from build123d import *

# Parameters (mm, degrees)
SKETCH1_W                 = 175
SKETCH1_H                 = 260
BOSS_EXTRUDE1_DEPTH       = 3
SKETCH3_W                 = 12.7
SKETCH3_H                 = 12.7
SKETCH3_W_2               = 8.7
SKETCH3_H_2               = 8.7
EXTRUDE_THIN1_DEPTH       = 328
MIRROR2_COPY_1_SKETCH_W   = 12.7
MIRROR2_COPY_1_SKETCH_H   = 12.7
MIRROR2_COPY_1_SKETCH_W_2 = 8.7
MIRROR2_COPY_1_SKETCH_H_2 = 8.7
MIRROR2_COPY_1_DEPTH      = 328
SKETCH5_W                 = 175
SKETCH5_H                 = 260
SKETCH5_W_2               = 171
SKETCH5_H_2               = 256
EXTRUDE_THIN2_DEPTH       = 83
SKETCH6_W                 = 175
SKETCH6_H                 = 260
BOSS_EXTRUDE2_DEPTH       = 2
SKETCH8_R                 = 22.5
CUT_EXTRUDE1_DEPTH        = 364.51100396
SKETCH9_R                 = 7.5
CUT_EXTRUDE2_DEPTH        = 3


with BuildPart() as part:
    # Sketch1 → Boss-Extrude1 (new body)
    with BuildSketch(Plane(origin=(0, 0, 0), x_dir=(1, 0, 0), z_dir=(0, 1, 0))):
        Rectangle(SKETCH1_W, SKETCH1_H)
    extrude(amount=BOSS_EXTRUDE1_DEPTH)

    # Sketch3 → Extrude-Thin1 (add)
    with BuildSketch(Plane(origin=(0, 3, 0), x_dir=(1, 0, 0), z_dir=(0, 1, 0))):
        with Locations((-81.15, 123.65)):
            Rectangle(SKETCH3_W, SKETCH3_H)
        with Locations((-81.15, 123.65)):
            Rectangle(SKETCH3_W_2, SKETCH3_H_2, mode=Mode.SUBTRACT)
    extrude_thin1 = extrude(amount=EXTRUDE_THIN1_DEPTH)

    # Mirror1: Extrude-Thin1 across plane
    add(extrude_thin1.mirror(Plane(origin=(0, 0, 0), x_dir=(0, 0, 1), z_dir=(1, 0, 0))))

    # Mirror2: Extrude-Thin1 across plane
    add(extrude_thin1.mirror(Plane.XY))

    # Mirror2 copy 1 sketch → Mirror2 copy 1 (add)
    with BuildSketch(Plane(origin=(0, 3, 0), x_dir=(-1, 0, 0), z_dir=(0, 1, 0))):
        with Locations((-81.15, 123.65)):
            Rectangle(MIRROR2_COPY_1_SKETCH_W, MIRROR2_COPY_1_SKETCH_H)
        with Locations((-81.15, 123.65)):
            Rectangle(MIRROR2_COPY_1_SKETCH_W_2, MIRROR2_COPY_1_SKETCH_H_2, mode=Mode.SUBTRACT)
    extrude(amount=MIRROR2_COPY_1_DEPTH)

    # Sketch5 → Extrude-Thin2 (add)
    with BuildSketch(Plane(origin=(0, 3, 0), x_dir=(1, 0, 0), z_dir=(0, 1, 0))):
        Rectangle(SKETCH5_W, SKETCH5_H)
        Rectangle(SKETCH5_W_2, SKETCH5_H_2, mode=Mode.SUBTRACT)
    extrude(amount=EXTRUDE_THIN2_DEPTH)

    # Sketch6 → Boss-Extrude2 (add)
    with BuildSketch(Plane(origin=(0, 86, 0), x_dir=(1, 0, 0), z_dir=(0, 1, 0))):
        Rectangle(SKETCH6_W, SKETCH6_H)
    extrude(amount=BOSS_EXTRUDE2_DEPTH)

    # Sketch8 → Cut-Extrude1 (cut, through all)
    with BuildSketch(Plane(origin=(0, 3, 0), x_dir=(1, 0, 0), z_dir=(0, 1, 0))):
        with Locations((0, -60)):
            Circle(SKETCH8_R)
        with BuildLine():
            ThreePointArc((22.5, 0), (0, -22.5), (-22.5, 0))
            Line((-22.5, 0), (-22.5, -60))
            ThreePointArc((-22.5, -60), (0, -37.5), (22.5, -60))
            Line((22.5, -60), (22.5, 0))
        make_face()
        Circle(SKETCH8_R)
    extrude(amount=CUT_EXTRUDE1_DEPTH, mode=Mode.SUBTRACT)

    # Sketch9 → Cut-Extrude2 (cut)
    with BuildSketch(Plane.XZ):
        with Locations((-15, -112.5)):
            Circle(SKETCH9_R)
        with BuildLine():
            Line((15, -105), (-15, -105))
            ThreePointArc((-15, -105), (-9.696699141, -107.196699141), (-7.5, -112.5))
            ThreePointArc((-7.5, -112.5), (-9.696699141, -117.803300859), (-15, -120))
            Line((-15, -120), (15, -120))
            ThreePointArc((15, -120), (7.5, -112.5), (15, -105))
        make_face()
        with Locations((15, -112.5)):
            Circle(SKETCH9_R)
    extrude(amount=-CUT_EXTRUDE2_DEPTH, mode=Mode.SUBTRACT)


solid = part.part
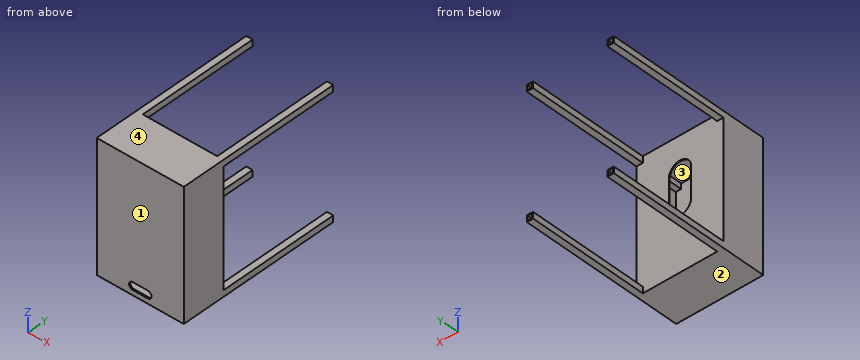
Geometry: final body of the model. Coordinates: model frame, mm. Face numbers are marked on the shaded views. Give positions to 0.01 mm unless a question says otherwise; leave off trailing zeros. Order: outer loops, then holes, each group sorted by start corner. A loop starts at its lowest first (then second) coordinate and runs counter-clockwise, first axis right, second up. Notation, with made-up numbers: (28.25, -33.75) -> (53.25, -33.75) arc R13 ccw to (53.25, -13.75) -> close; hole circle Ø1 at (-33, -2.75). An arc over 180 degrees is marked (long way). Write each question's results on one line, items separated by ' | '.
1) Cut plane D-D (z = 12). Output: boundary loops of the cut face in (x, y), and give its area (3 significant figures).
Geometry says:
outline: (-87.5, 0) -> (87.5, 0) -> (87.5, 88) -> (22.5, 88) -> (22.5, 86) -> (85.5, 86) -> (85.5, 3) -> (-85.5, 3) -> (-85.5, 86) -> (-22.5, 86) -> (-22.5, 88) -> (-87.5, 88) -> close | area: 1,120 mm²
2) Cut plane A-A (y = 110). Give the number of separate pieces and of enclosed holes in the cut face, and give its area (3 significant figures).
Geometry says:
separate pieces: 4 | enclosed holes: 4 | area: 342 mm²
3) Cut plane B-B (x = 0). Output: boundary loops of the cut face in (y, z), and give its area (3 significant figures).
Geometry says:
outline: (0, -130) -> (88, -130) -> (88, -22.5) -> (86, -22.5) -> (86, -128) -> (3, -128) -> (3, -120) -> (0, -120) -> close; (0, -105) -> (3, -105) -> (3, 128) -> (86, 128) -> (86, 82.5) -> (88, 82.5) -> (88, 130) -> (0, 130) -> close | area: 1,380 mm²
4) First-contact query: pin 1 Ø9.5 at (x, z) = (-81.5, 125.5) entering from -Y; pin 2 Ø2.5 at (x, z) = (79.5, -125) entering from +Y. Flat tips, straight axial feed; report the tip coordinate or a pass-through.
Geometry says:
pin 1: stops at y = 0 | pin 2: stops at y = 88
5) Draft query along Z for the marked faces 1, 2, 3 and 4. Return one class per face: released by +Z, released by -Z, zero draft, split by the parting line, or undercut.
Geometry says:
face 1: zero draft | face 2: released by -Z | face 3: undercut | face 4: released by +Z
6) Line query: line 1 along Z through (x, y) = (19, 16); line 2 along X through (y, z) = (38.5, -57); line 3 along Y through (x, z) = (-15.5, -18.5). Output: solid intervals per line, ascending.
Geometry says:
line 1: z = -130 to -128, 128 to 130 | line 2: x = -87.5 to -85.5, 85.5 to 87.5 | line 3: y = 0 to 3, 86 to 88
7) Cut plane C-C (x = 37.5). Output: boundary loops of the cut face in (y, z).
Geometry says:
outline: (0, -130) -> (88, -130) -> (88, 130) -> (0, 130) -> close; hole (3, -128) -> (86, -128) -> (86, 128) -> (3, 128) -> close
